from build123d import *

# Parameters (mm, degrees)
BOSS_EXTRUDE1_DEPTH = 24.892
CUT_EXTRUDE1_REACH  = 27.146
SKETCH2_W           = 16.764
SKETCH2_H           = 27.686
SKETCH3_R           = 3.302
SKETCH3_R_2         = 1.651
CUT_EXTRUDE2_DEPTH  = 24.892
CUT_EXTRUDE3_REACH  = 32.734
SKETCH4_W           = 3.81
SKETCH4_H           = 14.224
SKETCH4_W_2         = 3.302
FILLET1_R           = 2.54


with BuildPart() as part:
    # Sketch1 → Boss-Extrude1 (new body)
    with BuildSketch(Plane.XY):
        with BuildLine():
            Line((-14.605, 0), (14.605, 0))
            Line((14.605, 0), (14.605, 3.048))
            Line((14.605, 3.048), (10.541, 3.048))
            Line((10.541, 3.048), (10.541, 20.193))
            ThreePointArc((10.541, 20.193), (0, 30.734), (-10.541, 20.193))
            Line((-10.541, 20.193), (-10.541, 3.048))
            Line((-10.541, 3.048), (-14.605, 3.048))
            Line((-14.605, 3.048), (-14.605, 0))
        make_face()
    extrude(amount=BOSS_EXTRUDE1_DEPTH)

    # Sketch2 → Cut-Extrude1 (cut, up to next)
    with BuildSketch(Plane.ZY.offset(10.541), mode=Mode.PRIVATE) as cut_extrude1_sk1:
        with Locations((12.446, 16.891)):
            Rectangle(SKETCH2_W, SKETCH2_H)
    cut_extrude1_tool1 = extrude(cut_extrude1_sk1.sketch, amount=-CUT_EXTRUDE1_REACH, mode=Mode.PRIVATE) & part.part
    add(cut_extrude1_tool1.solids().sort_by_distance((-10.541, 16.891, 12.446))[0], mode=Mode.SUBTRACT)

    # Sketch3 → Cut-Extrude2 (cut)
    with BuildSketch(Plane(origin=(0, 0, 0), x_dir=(-1, 0, 0), z_dir=(0, 0, -1))):
        with Locations((-5.715, 21.59)):
            Circle(SKETCH3_R)
        with Locations((-6.731, 7.62)):
            Circle(SKETCH3_R_2)
        with Locations((0.127, 7.62)):
            Circle(SKETCH3_R_2)
        with Locations((6.477, 14.224)):
            Circle(SKETCH3_R_2)
    extrude(amount=-CUT_EXTRUDE2_DEPTH, mode=Mode.SUBTRACT)

    # Sketch4 → Cut-Extrude3 (cut, up to next)
    with BuildSketch(Plane.XZ, mode=Mode.PRIVATE) as cut_extrude3_sk1:
        with Locations((-7.321818594, 12.446)):
            Rectangle(SKETCH4_W, SKETCH4_H)
    cut_extrude3_tool1 = extrude(cut_extrude3_sk1.sketch, amount=-CUT_EXTRUDE3_REACH, mode=Mode.PRIVATE) & part.part
    add(cut_extrude3_tool1.solids().sort_by_distance((-7.321819, 0, 12.446))[0], mode=Mode.SUBTRACT)
    # Sketch4 → Cut-Extrude3 (cut, up to next)
    with BuildSketch(Plane.XZ, mode=Mode.PRIVATE) as cut_extrude3_sk2:
        with Locations((7.62, 12.446)):
            Rectangle(SKETCH4_W_2, SKETCH4_H)
    cut_extrude3_tool2 = extrude(cut_extrude3_sk2.sketch, amount=-CUT_EXTRUDE3_REACH, mode=Mode.PRIVATE) & part.part
    add(cut_extrude3_tool2.solids().sort_by_distance((7.62, 0, 12.446))[0], mode=Mode.SUBTRACT)

    # Fillet1
    fillet1_edges = [part.edges().sort_by_distance(p)[0] for p in [
        (-14.605, 3.048, 12.446),
        (14.605, 3.048, 12.446),
    ]]
    fillet(fillet1_edges, radius=FILLET1_R)


solid = part.part
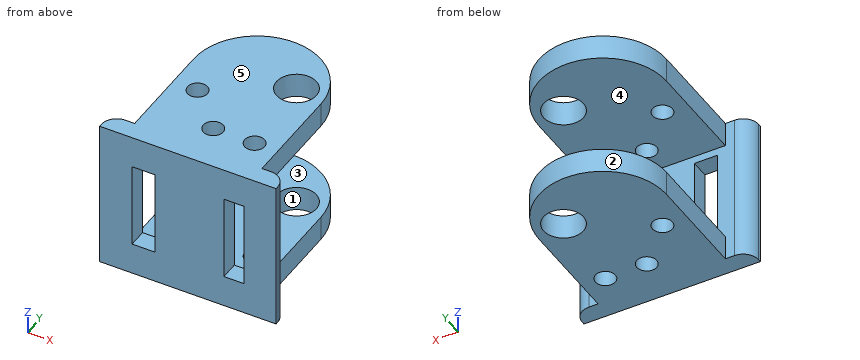
Model file for the job. Use its own axes, mm. Face numbers are marked on the shaded views. A direction names the side the tool comes from. Round coordinates to 2 decimals unless told otherwise and drop trailing zeros. Order: outer loops, then holes, each group sorted by start corner. A loop starts at its lowest first (then second) coordinate and runs counter-clockwise, first axis right, second up.
(1) Pin check, flat tips, straight feed: pin 1 (4.5 mm diameter, centred on y = 14.5, z = 1.5, fed in from +X); pin 2 (1.5 mm diameter, centred on y = 1.5, z = 12, fed in from +X); pin 3 (4.5 mm diameter, centred on y = 12.5, z = 23.5, fed in from -X). Stop position of each tip, or through.
(2) Band-saw the part on D-D (y = 25.5). List the corners of the cut face in (x, z), then the cut area to 3 significant figures.
(3) Band-saw the part on C-C (x = 0). List the corners of the cut face in (y, z).
(4) Drill centre lines: line 1 (Z direction, x = -6, y = 2.5); line 2 (Z direction, x = 0.5, y = 9.5); line 3 (Y direction, x = 6.25, z = 21.5). Where is each one in solid material? Low to high.
(5) Band-saw the part on B-B (y = 7.62). List the corners of the cut face in (x, z).
(6) 3-axis set-ups, long thin cutter, end or side, ignore diameter. For the marked faces 4 and 5: which of +Z, -Z, +X, -X, +Y, -Y reach the whole face in a straight line?
(7) Band-saw the part on A-A (z = 18). List the corners of the cut face in (x, y) (3 decimals), then the cut area to 3 significant figures.
(8) Pull direction Y, two halves, no side cores. Call the marked faces 1, 2 and 3: released by +Y, released by -Y, zero draft, split by the parting line, or undercut.
Verdict:
1. pin 1: stops at x = 10.54
1. pin 2: stops at x = 14.59
1. pin 3: stops at x = -10.54
2. outline: (-9.11, 0) - (9.11, 0) - (9.11, 4.06) - (-9.11, 4.06) - close; (-9.11, 20.83) - (9.11, 20.83) - (9.11, 24.89) - (-9.11, 24.89) - close
2. area: 148 mm2
3. outline: (0, 0) - (5.97, 0) - (5.97, 4.06) - (3.05, 4.06) - (3.05, 20.83) - (5.97, 20.83) - (5.97, 24.89) - (0, 24.89) - close; (9.27, 0) - (30.73, 0) - (30.73, 4.06) - (9.27, 4.06) - close; (9.27, 20.83) - (30.73, 20.83) - (30.73, 24.89) - (9.27, 24.89) - close
4. line 1: z = 0 to 5.33, 19.56 to 24.89
4. line 2: z = 0 to 4.06, 20.83 to 24.89
4. line 3: y = 0 to 6.04, 9.2 to 18.33, 24.85 to 28.68
5. outline: (-10.54, 0) - (-1.78, 0) - (-1.78, 4.06) - (-10.54, 4.06) - close; (-10.54, 20.83) - (-1.78, 20.83) - (-1.78, 24.89) - (-10.54, 24.89) - close; (1.52, 0) - (5.08, 0) - (5.08, 4.06) - (1.52, 4.06) - close; (1.52, 20.83) - (5.08, 20.83) - (5.08, 24.89) - (1.52, 24.89) - close; (8.38, 0) - (10.54, 0) - (10.54, 4.06) - (8.38, 4.06) - close; (8.38, 20.83) - (10.54, 20.83) - (10.54, 24.89) - (8.38, 24.89) - close
6. face 4: +X, -X, +Y
6. face 5: +Z, +X, -X, +Y, -Y
7. outline: (-14.605, 0) - (-9.227, 0) - (-9.227, 3.048) - (-12.065, 3.048) arc R2.54 ccw to (-14.605, 0.508) - close; (-5.417, 0) - (5.969, 0) - (5.969, 3.048) - (-5.417, 3.048) - close; (9.271, 0) - (14.605, 0) - (14.605, 0.508) arc R2.54 ccw to (12.065, 3.048) - (9.271, 3.048) - close
7. area: 64.6 mm2
8. face 1: undercut
8. face 2: released by +Y
8. face 3: zero draft
